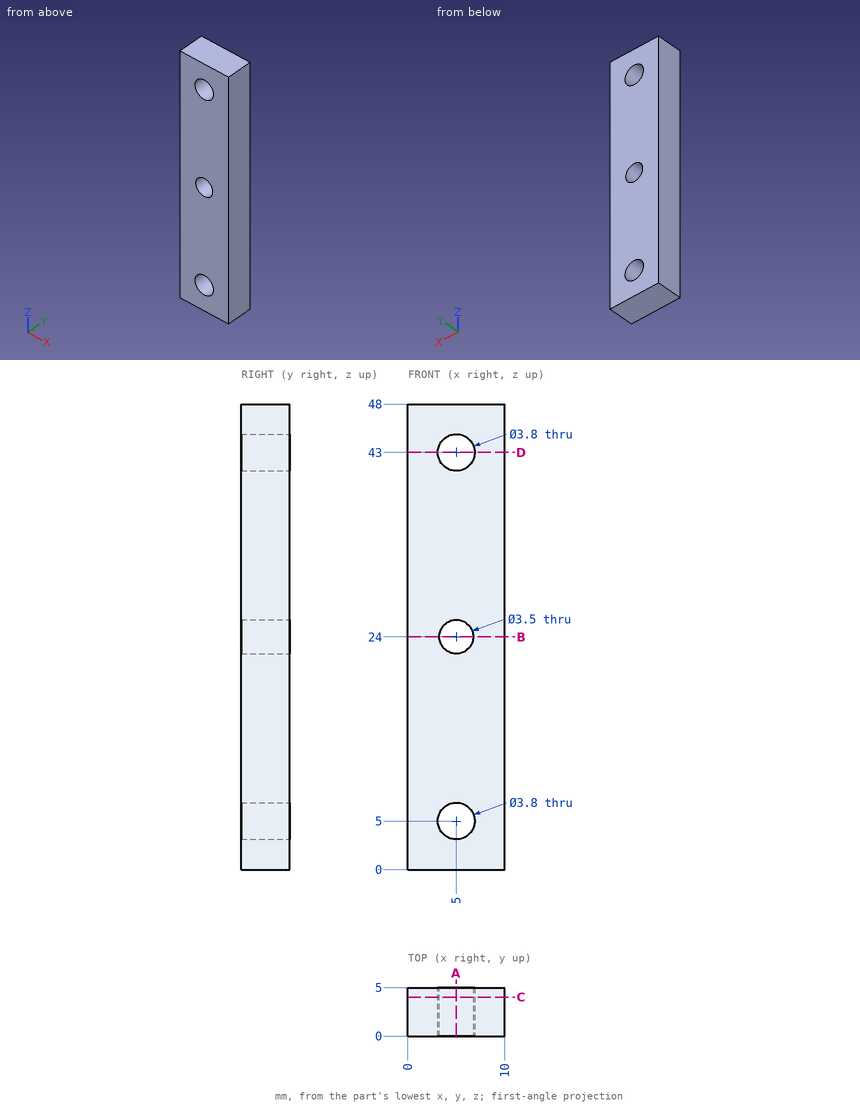
Geometry check sheet. Reference: drawing and pictorial views, mm from the part's lowest x, y, z. Round coordinates to 2 decimals unless told otherwise and drop trailing zeros. Loops run counter-clockwise (first coordinate to the right, second up) from the corner with the lowest first, then second, coordinate; pieces in that order, holes last. Notation, with made-up numbers: (33.5, 70) -> (42.5, 70) arc R7 cw to (42.5, 74) -> close; hole circle Ø4 at (7, 18.25). An arc over 180 degrees is marked (long way). Answer as a JSON object with one key per item and string values.
Q1. Section check C-C (y = 4). Record the boundary of the cut face in (x, z), then the cut area to 3 significant figures.
Data:
{"outline": "(0, 0) -> (10, 0) -> (10, 48) -> (0, 48) -> close; hole circle Ø3.8 at (5, 5); hole circle Ø3.8 at (5, 43); hole circle Ø3.5 at (5, 24)", "area": "448 mm2"}
Q2. Scan lines: line 1 (Z direction, x = 5, y = 1.15); line 2 (X direction, y = 1.75, z = 5); line 3 (Z direction, x = 6.5, y = 3.25). Record each from-to range of solid material in increasing order. Write a range as from..to.
Data:
{"line 1": "z = 0..3.1, 6.9..22.25, 25.75..41.1, 44.9..48", "line 2": "x = 0..3.1, 6.9..10", "line 3": "z = 0..3.83, 6.17..23.1, 24.9..41.83, 44.17..48"}
Q3. Section check D-D (z = 43). Record the boundary of the cut face in (x, y).
Data:
{"outline": "(0, 0) -> (3.1, 0) -> (3.1, 5) -> (0, 5) -> close; (6.9, 0) -> (10, 0) -> (10, 5) -> (6.9, 5) -> close"}
Q4. Go/stop test with a flat-tipped pin: P1, Ø3, axis at x = 5, z = 5, coming from the -Y side. Record where the tip stops, or that it passes through.
Data:
{"P1": "passes through"}
Q5. Section check B-B (z = 24). Record the boundary of the cut face in (x, y).
Data:
{"outline": "(0, 0) -> (3.25, 0) -> (3.25, 5) -> (0, 5) -> close; (6.75, 0) -> (10, 0) -> (10, 5) -> (6.75, 5) -> close"}
Q6. Section check A-A (x = 5). Record the boundary of the cut face in (y, z).
Data:
{"outline": "(0, 0) -> (5, 0) -> (5, 3.1) -> (0, 3.1) -> close; (0, 6.9) -> (5, 6.9) -> (5, 22.25) -> (0, 22.25) -> close; (0, 25.75) -> (5, 25.75) -> (5, 41.1) -> (0, 41.1) -> close; (0, 44.9) -> (5, 44.9) -> (5, 48) -> (0, 48) -> close"}
